Here's the drawing with two shaded views (mm, measured from the low corner). I have some questions. Coordinates: 2 decimals unless noted, no trailing zeros. Loops run counter-clockwise (first coordinate to the right, second up) from the corner with the lowest first, then second, coordinate; pieces in that order, holes last. Notation, with made-up numbers: (4.25, -6.5) - (45.25, -6.5) arc R12 cw to (45.25, 5.5) - close; hole circle Ø7 at (78.25, 29). An arc over 180 degrees is marked (long way). One line per item, written item: value. Start each with the question number.
(1) If we section it at B-B on z = 2.9: Write out the boundary of the cut face in (x, y).
(2) If we section it at D-D on y = 10: Write out the boundary of the cut face in (x, z).
(3) If we mould it in two halves opening along Y, with no side actions, what happens to the marked faces 1, 2 and 3? For each: pulls with the +Y half, pulls with the -Y half, needs draft (parallel to the pull), parting line crosses it, or undercut.
(4) I'm going to push flat-ended pins straight in: P1, Ø1.5, axis at x = 30, y = 44.5, coming from the -Z side; P2, Ø2.5, axis at x = 10, y = 55, coming from the +Z side. Where does each tip first touch, or does it pass through?
(5) If I drill on line 1 along X through (y, z) = (10, 1.5); line 2 along Y through (x, z) = (20, 1.3); line 3 along Y through (x, z) = (30, 2), over which ranges is the centre line in solid material (lowest first)? Write a range as from..to.
(6) If we section it at C-C on x = 20: Write out the boundary of the cut face in (y, z), then the cut area to 3 significant figures.
(7) If we section it at A-A on y = 25: Write out the boundary of the cut face in (x, z).
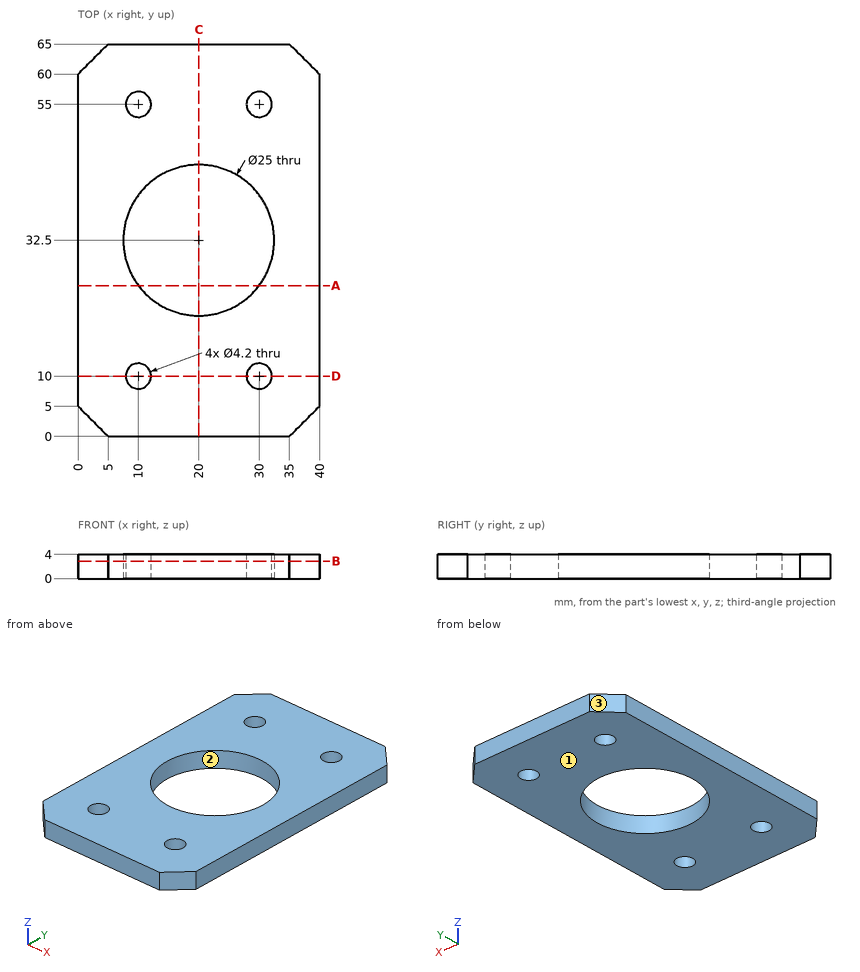
Values:
1. outline: (0, 5) - (5, 0) - (35, 0) - (40, 5) - (40, 60) - (35, 65) - (5, 65) - (0, 60) - close; hole circle Ø25 at (20, 32.5); hole circle Ø4.2 at (10, 10); hole circle Ø4.2 at (10, 55); hole circle Ø4.2 at (30, 10); hole circle Ø4.2 at (30, 55)
2. outline: (0, 0) - (7.9, 0) - (7.9, 4) - (0, 4) - close; (12.1, 0) - (27.9, 0) - (27.9, 4) - (12.1, 4) - close; (32.1, 0) - (40, 0) - (40, 4) - (32.1, 4) - close
3. face 1: needs draft
3. face 2: undercut
3. face 3: pulls with the +Y half
4. P1: stops at z = 0
4. P2: passes through
5. line 1: x = 0..7.9, 12.1..27.9, 32.1..40
5. line 2: y = 0..20, 45..65
5. line 3: y = 0..7.9, 12.1..25, 40..52.9, 57.1..65
6. outline: (0, 0) - (20, 0) - (20, 4) - (0, 4) - close; (45, 0) - (65, 0) - (65, 4) - (45, 4) - close
6. area: 160 mm2
7. outline: (0, 0) - (10, 0) - (10, 4) - (0, 4) - close; (30, 0) - (40, 0) - (40, 4) - (30, 4) - close
